```python
from build123d import *

# Parameters (mm, degrees)
SKETCH2_W          = 50.8
SKETCH2_H          = 127
BASE_DEPTH         = 5.334
SKETCH3_W          = 19.05
SKETCH3_H          = 5.334
TABS_DEPTH         = 5.334
SKETCH4_W          = 12.7
SKETCH4_H          = 2.4638
MOUNT_POINTS_DEPTH = 142.849847064


with BuildPart() as part:
    # Sketch2 → Base (new body)
    with BuildSketch(Plane(origin=(0, 0, 0), x_dir=(1, 0, 0), z_dir=(0, 1, 0))):
        with Locations((25.4, 63.5)):
            Rectangle(SKETCH2_W, SKETCH2_H)
    extrude(amount=BASE_DEPTH)

    # Sketch3 → Tabs (add)
    with BuildSketch(Plane.XY):
        with Locations((25.4, 2.667)):
            Rectangle(SKETCH3_W, SKETCH3_H)
    tabs = extrude(amount=TABS_DEPTH)

    # Tabs Mirror: Tabs across plane
    add(tabs.mirror(Plane.XY.offset(-63.5)))

    # Sketch4 → Mount Points (cut, through all)
    with BuildSketch(Plane.XZ):
        with Locations((11.75, -35.145453499)):
            Rectangle(SKETCH4_W, SKETCH4_H)
        with Locations((39.05, -35.145453499)):
            Rectangle(SKETCH4_W, SKETCH4_H)
        with Locations((11.75, -88.409253499)):
            Rectangle(SKETCH4_W, SKETCH4_H)
        with Locations((39.05, -88.409253499)):
            Rectangle(SKETCH4_W, SKETCH4_H)
    extrude(amount=-MOUNT_POINTS_DEPTH, mode=Mode.SUBTRACT)


solid = part.part
```
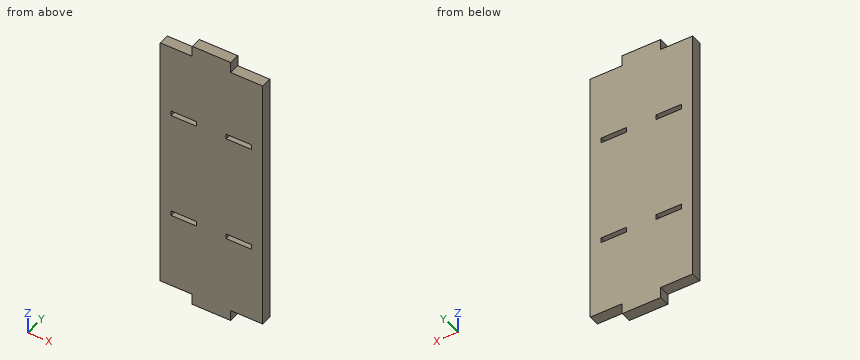
Model file for the job. Use its own axes, mm. Coordinates: 2 decimals unless noted, no trailing zeros. Loops run counter-clockwise (first coordinate to the right, second up) from the corner with the lowest first, then second, coordinate; pieces in that order, holes last. Notation, with made-up numbers: (-18, 25) -> (31, 25) arc R19 cw to (31, 46) -> close; hole circle Ø3 at (-18.75, 14). An arc over 180 degrees is marked (long way). Answer as a JSON object with one key per item and string values.
Q1. Cut at B-B (y = 4.1). List the corners of the cut face in (x, z) (3 decimals).
Report:
{"outline": "(0, -127) -> (15.875, -127) -> (15.875, -132.334) -> (34.925, -132.334) -> (34.925, -127) -> (50.8, -127) -> (50.8, 0) -> (34.925, 0) -> (34.925, 5.334) -> (15.875, 5.334) -> (15.875, 0) -> (0, 0) -> close; hole (5.4, -89.641) -> (18.1, -89.641) -> (18.1, -87.177) -> (5.4, -87.177) -> close; hole (5.4, -36.377) -> (18.1, -36.377) -> (18.1, -33.914) -> (5.4, -33.914) -> close; hole (32.7, -89.641) -> (45.4, -89.641) -> (45.4, -87.177) -> (32.7, -87.177) -> close; hole (32.7, -36.377) -> (45.4, -36.377) -> (45.4, -33.914) -> (32.7, -33.914) -> close"}
Q2. Flat gauge pins, fed straight in: P1, Ø2.5, axis at x = 37, y = 2, coming from the -Z side; P2, Ø2.5, axis at y = 2.5, z = -130, coming from the -X side (3 decimals); P3, Ø3, axis at x = 42, y = 2, coming from the +Z side. Where does each tip first touch, or does it go through?
Report:
{"P1": "stops at z = -127", "P2": "stops at x = 15.875", "P3": "stops at z = 0"}
Q3. Cut at A-A (x = 10). List the corners of the cut face in (y, z), and give its area (3 significant figures).
Report:
{"outline": "(0, -127) -> (5.33, -127) -> (5.33, -89.64) -> (0, -89.64) -> close; (0, -87.18) -> (5.33, -87.18) -> (5.33, -36.38) -> (0, -36.38) -> close; (0, -33.91) -> (5.33, -33.91) -> (5.33, 0) -> (0, 0) -> close", "area": "651 mm2"}
Q4. Probe probe 1 along Z at (x, y) = (38.5, 3); probe 2 along Z at (x, y) = (45.5, 1.65). List the from-to ranges inside material, lowest first.
Report:
{"probe 1": "z = -127 to -89.64, -87.18 to -36.38, -33.91 to 0", "probe 2": "z = -127 to 0"}
